```python
from build123d import *

# Parameters (mm, degrees)
F1_DEPTH = 50
F2_DEPTH = 25
F3_R     = 5
F4_R     = 5
F5_R     = 5
F6_R     = 5


with BuildPart() as f1:
    # F0 (on Front) → F1 (new body)
    with BuildSketch(Plane.XZ):
        Polygon((268, 2), (2, 2), (2, 150), (0, 150), (0, 0), (270, 0), (270, 150), (268, 150), align=None)
    extrude(amount=F1_DEPTH)

    # F0 (on Front) → F2 (join)
    with BuildSketch(Plane.XZ):
        Polygon((268, 2), (2, 2), (2, 150), (0, 150), (0, 0), (270, 0), (270, 150), (268, 150), align=None)
    extrude(amount=F2_DEPTH)

    # F3
    f3_edges = [f1.edges().sort_by_distance(p)[0] for p in [
        (0, -25, 0),
    ]]
    fillet(f3_edges, radius=F3_R)

    # F4
    f4_edges = [f1.edges().sort_by_distance(p)[0] for p in [
        (2, -25, 2),
    ]]
    fillet(f4_edges, radius=F4_R)

    # F5
    f5_edges = [f1.edges().sort_by_distance(p)[0] for p in [
        (270, -25, 0),
    ]]
    fillet(f5_edges, radius=F5_R)

    # F6
    f6_edges = [f1.edges().sort_by_distance(p)[0] for p in [
        (268, -25, 2),
    ]]
    fillet(f6_edges, radius=F6_R)


solid = f1.part
```
Input: part model. Units: mm. Frame: model coordinates. A direction names the side the tool comes from. Round coordinates to 2 decimals unless told otherwise and drop trailing zeros. Write each loop counter-clockwise with the first axis right and the second up, starting at its lowest first coordinate (ties: lowest second). Pieces come first, ordered by that corner, then holes. Notation, with made-up numbers: (2.5, -19) - (48.5, -19) arc R4 ccw to (48.5, -12) - close; hole circle Ø2 at (87, -6). An arc over 180 degrees is marked (long way). Write item = value, one per line.
(1) Access query for faces 5 (the cylindrical face through (268, -25, 1)), 6 (the cylindrical face through (3, -25, 4)). Directions: +Z, -Z, +X, -X, +Y, -Y. A direction counts if a zero-diameter tool reaches every point of the face in a straight line with its end or side. Return the directions, or none.
Geometry check:
face_5 = -Z, +X, +Y, -Y
face_6 = +Z, +Y, -Y
(2) Section query A-A on z = 139.5. Output: boundary loops of the cut face in (x, y).
Geometry check:
outline = (0, -50) - (2, -50) - (2, 0) - (0, 0) - close; (268, -50) - (270, -50) - (270, 0) - (268, 0) - close
(3) Section query C-C on x = 250.5. Output: boundary loops of the cut face in (y, z), then the cut area to 3 significant figures.
Geometry check:
outline = (-50, 0) - (0, 0) - (0, 2) - (-50, 2) - close
area = 100 mm^2
(4) Material intervals for probe 1 along X at (y, z) = (-41.5, 117); probe 2 along Z at (x, y) = (183, -26), sorted ascending.
Geometry check:
probe_1 = 0 to 2, 268 to 270
probe_2 = 0 to 2
(5) Pull-direction query (X, two-part tool) for faces 1 (the flat face through (270, -25, 76)), 2 (the flat face through (0, -25, 79)), 3 (the flat face through (137, -25, 2)), 4 (the flat face through (268, -25, 80)); classes: +X half, -X half, draft (parallel to the pull), parting line (faces both ways), or undercut.
Geometry check:
face_1 = +X half
face_2 = -X half
face_3 = undercut
face_4 = undercut
(6) Section query B-B on y = -31.5. Output: boundary loops of the cut face in (x, z).
Geometry check:
outline = (0, 5) arc R5 ccw to (5, 0) - (265, 0) arc R5 ccw to (270, 5) - (270, 150) - (268, 150) - (268, 7) arc R5 cw to (263, 2) - (7, 2) arc R5 cw to (2, 7) - (2, 150) - (0, 150) - close
(7) Contact query for a flat-ended pin moving along its axis: pin 1 Ø2 at (x, y) = (113.5, -17.5) entering from +Z. Output: stop coordinate, or through.
Geometry check:
pin_1 = 2
